Part print with two shaded views. Sizes in mm from the minimum x, y, z corner. Coordinates: 2 decimals unless noted, no trailing zeros. Loops run counter-clockwise (first coordinate to the right, second up) from the corner with the lowest first, then second, coordinate; pieces in that order, holes last.
(1) Flat gauge pins, fed straight in: P1, Ø6, axis at x = 668, y = 94, coming from the -Z side; P2, Ø6, axis at x = 672.5, y = 114, coming from the +Z side; P3, Ø16, axis at y = 209.5, z = 457, coming from the -X side. Where does each tip first touch, or does it go through?
(2) Slice it at B-B (x = 195). Give the cut face in (y, z), and give its area (3 significant figures).
(3) Wall check: L1, parallel to X at y = 205.5, z = 62; L2, parallel to Z at x = 65, y = 199.5; L3, parallel to X at y = 188, z = 528.5. Give the ranges that are in metal, low to high.
(4) Slice it at A-A (z = 498). Give the cut face in (x, y), and give its area (3 significant figures).
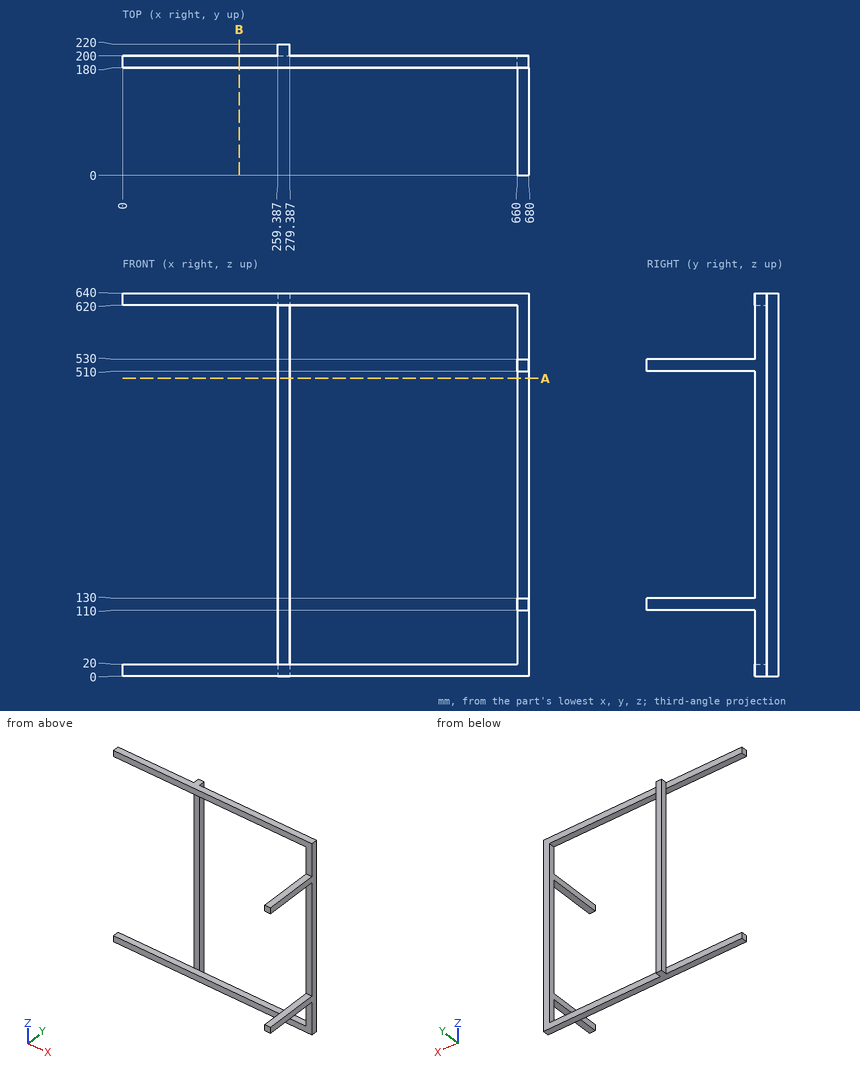
Response values:
1. P1: stops at z = 110
1. P2: stops at z = 530
1. P3: stops at x = 259.39
2. outline: (180, 0) - (200, 0) - (200, 20) - (180, 20) - close; (180, 620) - (200, 620) - (200, 640) - (180, 640) - close
2. area: 800 mm2
3. L1: x = 259.39 to 279.39
3. L2: z = 0 to 20, 620 to 640
3. L3: x = 660 to 680
4. outline: (259.39, 200) - (279.39, 200) - (279.39, 220) - (259.39, 220) - close; (660, 180) - (680, 180) - (680, 200) - (660, 200) - close
4. area: 800 mm2
